from build123d import *

# Parameters (mm, degrees)
F1_DEPTH = 5.08


with BuildPart() as f1:
    # F0 (on Top) → F1 (new body)
    with BuildSketch(Plane.XY):
        Polygon((-4.270472, 55.757098), (-55.070472, 55.757098), (-55.070472, 30.357098), (-47.450472, 30.357098), (-47.450472, 10.037098), (-55.070472, 10.037098), (-55.070472, -25.522902), (-47.450472, -25.522902), (-47.450472, -45.842902), (-55.070472, -45.842902), (-55.070472, -71.242902), (-4.270472, -71.242902), (-4.270472, -45.842902), (-11.890472, -45.842902), (-11.890472, -25.522902), (-4.270472, -25.522902), (-4.270472, 10.037098), (-11.890472, 10.037098), (-11.890472, 30.357098), (-4.270472, 30.357098), align=None)
        Polygon((-49.990472, -51.771179), (-42.370472, -51.771179), (-32.210472, -51.892635), (-27.130472, -51.953363), (-16.970472, -52.07482), (-9.350472, -52.07482), (-9.350472, -65.435126), (-27.130472, -65.435126), (-32.210472, -65.435126), (-49.990472, -65.435126), align=None, mode=Mode.SUBTRACT)
        with BuildLine():
            Line((-16.970472, -45.842902), (-42.370472, -45.842902))
            ThreePointArc((-42.370472, -45.842902), (-39.50785, -37.810717), (-32.210472, -33.399494))
            Line((-32.210472, -33.399494), (-32.210472, -40.014148))
            ThreePointArc((-32.210472, -40.014148), (-29.670472, -44.004216), (-27.130472, -40.014148))
            Line((-27.130472, -40.014148), (-27.130472, -33.399494))
            ThreePointArc((-27.130472, -33.399494), (-19.833094, -37.810717), (-16.970472, -45.842902))
        make_face(mode=Mode.SUBTRACT)
        with BuildLine():
            Line((-49.990472, 48.734743), (-42.370472, 48.734743))
            Line((-42.370472, 48.734743), (-32.210472, 48.734743))
            Line((-32.210472, 48.734743), (-32.210472, -26.999166))
            ThreePointArc((-32.210472, -26.999166), (-37.999229, -29.353544), (-42.370472, -33.81953))
            Line((-42.370472, -33.81953), (-42.370472, -15.24))
            Line((-42.370472, -15.24), (-50.352603, -15.24))
            Line((-50.352603, -15.24), (-50.352603, 0))
            Line((-50.352603, 0), (-42.370472, 0))
            Line((-42.370472, 0), (-42.370472, 36.892656))
            Line((-42.370472, 36.892656), (-49.990472, 36.892656))
            Line((-49.990472, 36.892656), (-49.990472, 48.734743))
        make_face(mode=Mode.SUBTRACT)
        with BuildLine():
            Line((-27.130472, -26.922115), (-27.130472, 49.038388))
            Line((-27.130472, 49.038388), (-16.970472, 49.038388))
            Line((-16.970472, 49.038388), (-9.350472, 49.038388))
            Line((-9.350472, 49.038388), (-9.350472, 36.892656))
            Line((-9.350472, 36.892656), (-16.970472, 36.892656))
            Line((-16.970472, 36.892656), (-16.970472, 0))
            Line((-16.970472, 0), (-9.046003, 0))
            Line((-9.046003, 0), (-9.046003, -15.24))
            Line((-9.046003, -15.24), (-16.970472, -15.24))
            Line((-16.970472, -15.24), (-16.970472, -33.142902))
            ThreePointArc((-16.970472, -33.142902), (-21.422603, -29.007051), (-27.130472, -26.922115))
        make_face(mode=Mode.SUBTRACT)
    extrude(amount=F1_DEPTH)


solid = f1.part
Geometry: final body of the model. Coordinates: model frame, mm. A direction names the side the tool comes from. Coordinates: 2 decimals unless noted, no trailing zeros. Order: outer loops, then holes, each group sorted by start corner. A loop starts at its lowest first (then second) coordinate and runs counter-clockwise, first axis right, second up.
(1) First-contact query: pin 1 (1.5 mm diameter, centred on y = 22, z = 2.5, fed in from -X). Flat tip, straight axial feed; report the tip coordinate or a pass-through.
(2) Section query A-A (y = 40.5). Return the cut outline in (x, z), plus the area to 3 significant figures.
(3) Draft query along Y for faces 1 (the face through (-29, 55.757, 3)), 2 (the face through (-46, 0, 3)), 3 (the face through (-55.07, -58, 3)). Return one class per face: pulls with the +Y half, pulls with the -Y half, needs draft (parallel to the pull), parting line crosses it, or undercut.
(4) Section query D-D (x = -20). Return the cut outline in (y, z).
(5) Section query C-C (y = -17.5). Return the cut outline in (x, z), plus the area to 3 significant figures.
(6) Access query for faces 4 (the face through (-8, -45.843, 3)), 5 (the face through (-47.45, -36, 3)), 6 (the face through (-9.35, 43, 3)). Directions: +Z, -Z, +X, -X, +Y, -Y. A direction counts if a zero-diameter tool reaches every point of the face in a straight line with its end or side. Return the directions, or none.
(7) Material intervals for probe 1 along X at (y, z) = (20, 3.5); probe 2 along X at (y, z) = (1.5, 2); probe 3 along Y at (x, z) = (-43.5, 1), sorted ascending.
(8) Section query B-B (x = -44). Return the cut outline in (y, z).
Solution:
1. pin 1: stops at x = -47.45
2. outline: (-55.07, 0) - (-49.99, 0) - (-49.99, 5.08) - (-55.07, 5.08) - close; (-32.21, 0) - (-27.13, 0) - (-27.13, 5.08) - (-32.21, 5.08) - close; (-9.35, 0) - (-4.27, 0) - (-4.27, 5.08) - (-9.35, 5.08) - close
2. area: 77.4 mm2
3. face 1: pulls with the +Y half
3. face 2: undercut
3. face 3: needs draft
4. outline: (-71.24, 0) - (-65.44, 0) - (-65.44, 5.08) - (-71.24, 5.08) - close; (-52.04, 0) - (-45.84, 0) - (-45.84, 5.08) - (-52.04, 5.08) - close; (-37.61, 0) - (-29.99, 0) - (-29.99, 5.08) - (-37.61, 5.08) - close; (49.04, 0) - (55.76, 0) - (55.76, 5.08) - (49.04, 5.08) - close
5. outline: (-55.07, 0) - (-42.37, 0) - (-42.37, 5.08) - (-55.07, 5.08) - close; (-32.21, 0) - (-27.13, 0) - (-27.13, 5.08) - (-32.21, 5.08) - close; (-16.97, 0) - (-4.27, 0) - (-4.27, 5.08) - (-16.97, 5.08) - close
5. area: 155 mm2
6. face 4: +Z, -Z, +X
6. face 5: +Z, -Z, -X
6. face 6: +Z, -Z
7. probe 1: x = -47.45 to -42.37, -32.21 to -27.13, -16.97 to -11.89
7. probe 2: x = -55.07 to -42.37, -32.21 to -27.13, -16.97 to -4.27
7. probe 3: y = -71.24 to -65.44, -51.77 to -15.24, 0 to 36.89, 48.73 to 55.76
8. outline: (-71.24, 0) - (-65.44, 0) - (-65.44, 5.08) - (-71.24, 5.08) - close; (-51.77, 0) - (-15.24, 0) - (-15.24, 5.08) - (-51.77, 5.08) - close; (0, 0) - (36.89, 0) - (36.89, 5.08) - (0, 5.08) - close; (48.73, 0) - (55.76, 0) - (55.76, 5.08) - (48.73, 5.08) - close
